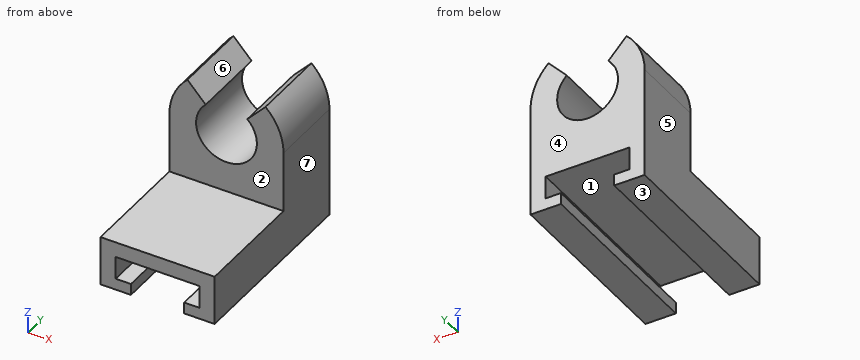
```python
from build123d import *

# Parameters (mm, degrees)
BOSS_EXTRUDE2_DEPTH = 25
BOSS_EXTRUDE3_DEPTH = 10


with BuildPart() as part:
    # Sketch1 → Boss-Extrude2 (new body)
    with BuildSketch(Plane(origin=(0, 0, 0), x_dir=(1, 0, 0), z_dir=(0, 1, 0))):
        Polygon((0, 0), (15, 0), (15, 6.5), (11, 6.5), (11, 5), (13, 5), (13, 2), (2, 2), (2, 5), (4, 5), (4, 6.5), (0, 6.5), align=None)
    extrude(amount=BOSS_EXTRUDE2_DEPTH)

    # Sketch2 → Boss-Extrude3 (add)
    with BuildSketch(Plane(origin=(0, 25, 0), x_dir=(1, 0, 0), z_dir=(0, 1, 0))):
        with BuildLine():
            Line((15, -8), (15, 0))
            Line((15, 0), (0, 0))
            Line((0, 0), (0, -8))
            ThreePointArc((0, -8), (0.618078448, -10.981468724), (2.370441533, -13.471529031))
            Line((2.370441533, -13.471529031), (4.764235484, -10.918148817))
            ThreePointArc((4.764235484, -10.918148817), (7.5, -4), (10.235764516, -10.918148817))
            Line((10.235764516, -10.918148817), (12.629558467, -13.471529031))
            ThreePointArc((12.629558467, -13.471529031), (14.381921552, -10.981468724), (15, -8))
        make_face()
    extrude(amount=-BOSS_EXTRUDE3_DEPTH)


solid = part.part
```
Could you check a few things on this model? Use its own coordinates, in mm. Face numbers are marked on the shaded views. A direction names the side the tool comes from. Round coordinates to 2 decimals unless told otherwise and drop trailing zeros. Loops run counter-clockwise (first coordinate to the right, second up) from the corner with the lowest first, then second, coordinate; pieces in that order, holes last. Notation, with made-up numbers: (-31.5, 52.5) -> (-11.5, 52.5) arc R22 ccw to (-11.5, 77.5) -> close; hole circle Ø11 at (60.5, 54). An arc over 180 degrees is marked (long way). Put each result on its own line as item: value.
Q1. Which directions (+Z, -Z, +X, -X, +Y, -Y) give clear straight access to the entire face, cutting with the end or side of a thin tool? Please do the marked faces 1, 2 and 3.
Checks:
face 1: +Y, -Y
face 2: +Z, +X, -X, -Y
face 3: -Z, +X, -X, +Y, -Y
Q2. I want a section at A-A on y = 4.5. Write out the boundary of the cut face in (x, z).
Checks:
outline: (0, -6.5) -> (4, -6.5) -> (4, -5) -> (2, -5) -> (2, -2) -> (13, -2) -> (13, -5) -> (11, -5) -> (11, -6.5) -> (15, -6.5) -> (15, 0) -> (0, 0) -> close
Q3. I want a section at B-B on x = 2.75. Write out the boundary of the cut face in (y, z), and give its area (3 significant figures).
Checks:
outline: (0, -6.5) -> (25, -6.5) -> (25, -5) -> (0, -5) -> close; (0, -2) -> (25, -2) -> (25, 13.07) -> (15, 13.07) -> (15, 0) -> (0, 0) -> close
area: 218 mm2
Q4. Please list where these lines run through material, in increasing order: line 1 (X direction, y = 19.25, z = 8); line 2 (Z direction, x = 3.5, y = 7.5); line 3 (X direction, y = 2.5, z = -4.5). Write a range as from..to.
Checks:
line 1: 0..3.5, 11.5..15
line 2: -6.5..-5, -2..0
line 3: 0..2, 13..15
Q5. For pin 1 Ø10 at (y, z) = (4, 6) entering from +X; pin 2 Ø2 at (x, y) = (11.5, 16.5) entering from +Z; pin 3 Ø2 at (x, y) = (2, 16.5) entering from +Z; pin 4 Ø8 at (x, z) = (7.5, 7.5) entering from -Y, each with a flat end and sliding along its axis, tell me the tip position at first contact or that it passes through.
Checks:
pin 1: through
pin 2: z = 13.33
pin 3: z = 13.47
pin 4: y = 15
Q6. Thinking about a two-plate mould opening in X: for the marked faces 4, 5, 6 and 7, which applies, pulls with the +X half, pulls with the -X half, needs draft (parallel to the pull), parting line crosses it, or undercut?
Checks:
face 4: needs draft
face 5: pulls with the -X half
face 6: undercut
face 7: pulls with the +X half
Q7. I want a section at C-C on z = 12. Write out the boundary of the cut face in (x, y), and give its area (3 significant figures).
Checks:
outline: (1.16, 15) -> (3.75, 15) -> (3.75, 25) -> (1.16, 25) -> close; (11.25, 15) -> (13.84, 15) -> (13.84, 25) -> (11.25, 25) -> close
area: 51.9 mm2
Q8. I want a section at D-D on x = 7.5. Write out the boundary of the cut face in (y, z), and give its area (3 significant figures).
Checks:
outline: (0, -2) -> (25, -2) -> (25, 4) -> (15, 4) -> (15, 0) -> (0, 0) -> close
area: 90.0 mm2
